Build history of the part. All positions in model axes, mm. Round coordinates to 2 decimals unless told otherwise and drop trailing zeros. Write each loop counter-clockwise with the first axis right and the second up, starting at its lowest first coordinate (ties: lowest second). Pieces come first, ordered by that corner, then holes.
1) Wall check: probe 1 along X at (y, z) = (30, 2); probe 2 along Y at (x, z) = (133.5, 4.25); probe 3 along X at (y, z) = (9.5, 0.5). Give the ranges that are in metal, low to high.
2) Flat gauge pins, fed straight in: pin 1 (9 mm diameter, centred on x = 127, y = 31.75, fed in from -Z); pin 2 (2 mm diameter, centred on x = 98.425, z = 5.08, fed in from +Y). Where does each tip first touch, or does it go through?
3) Pull direction Y, two halves, no side cores. Call faces 1 (the cylindrical face through (23.93, 51.16, 4.7)), 2 (the flat face through (69, 0, 5)), 3 (the cylindrical face through (98.501, 57.061, 6.806)): +Y half, -Y half, draft (parallel to the pull), parting line (faces both ways), or undercut.
4) Saw through at C-C (x = 25.4). Write the cut outline in (y, z) (3 decimals).
5) Saw through at B-B (z = 2). Write the cut outline in (x, y) (3 decimals).
6) Saw through at D-D (x = 94.5). Write the cut outline in (y, z) (3 decimals).
7) Saw through at A-A (x = 78.74). Write the cut outline in (y, z) (3 decimals).
from build123d import *

# Parameters (mm, degrees)
SKETCH1_W                   = 139.7
SKETCH1_H                   = 63.5
BOSS_EXTRUDE1_DEPTH         = 9.525
F_5_8_18_TAPPED_HOLE1_D     = 14.68374
F_1_4_0_25_DIAMETER_HOLE1_D = 6.35
F_8_32_TAPPED_HOLE1_D       = 3.4544
F_8_32_TAPPED_HOLE1_DEPTH   = 12.7
F_8_32_TAPPED_HOLE1_TIP     = 1.037806461
SKETCH9_R                   = 3.175
CUT_EXTRUDE1_DEPTH          = 10.525


with BuildPart() as part:
    # Sketch1 → Boss-Extrude1 (new body)
    with BuildSketch(Plane.XY):
        with Locations((69.85, 31.75)):
            Rectangle(SKETCH1_W, SKETCH1_H)
    extrude(amount=BOSS_EXTRUDE1_DEPTH)

    # 5/8-18 Tapped Hole1 (through all)
    with Locations(Plane.XY.offset(9.525)):
        with Locations((127, 31.75)):
            Hole(F_5_8_18_TAPPED_HOLE1_D / 2)

    # 1/4 (0.25) Diameter Hole1 (through all)
    with Locations(Plane(origin=(25.4, 53.975, 9.525), x_dir=(1, 0, 0), z_dir=(0, 0, 1))):
        with Locations((0, 0), (0, -44.45)):
            Hole(F_1_4_0_25_DIAMETER_HOLE1_D / 2)

    # #8-32 Tapped Hole1
    with Locations(Plane(origin=(98.425, 63.5, 5.08), x_dir=(0, 0, 1), z_dir=(0, 1, 0))):
        with Locations((0, 0)):
            Hole(F_8_32_TAPPED_HOLE1_D / 2, depth=F_8_32_TAPPED_HOLE1_DEPTH)
            with Locations((0, 0, -(F_8_32_TAPPED_HOLE1_DEPTH + F_8_32_TAPPED_HOLE1_TIP / 2))):  # 118° drill point
                Cone(0, F_8_32_TAPPED_HOLE1_D / 2, F_8_32_TAPPED_HOLE1_TIP, mode=Mode.SUBTRACT)

    # Sketch9 → Cut-Extrude1 (cut, through all)
    with BuildSketch(Plane.XY.offset(9.525)):
        with Locations((95.25, 31.75)):
            Circle(SKETCH9_R)
        with Locations((78.74, 31.75)):
            Circle(SKETCH9_R)
    extrude(amount=-CUT_EXTRUDE1_DEPTH, mode=Mode.SUBTRACT)


solid = part.part
Evaluation:
1. probe 1: x = 0 to 76.09, 81.39 to 92.6, 97.9 to 119.87, 134.13 to 139.7
1. probe 2: y = 0 to 28.34, 35.16 to 63.5
1. probe 3: x = 0 to 22.23, 28.57 to 139.7
2. pin 1: passes through
2. pin 2: stops at y = 50.36
3. face 1: undercut
3. face 2: -Y half
3. face 3: draft
4. outline: (0, 0) - (6.35, 0) - (6.35, 9.525) - (0, 9.525) - close; (12.7, 0) - (50.8, 0) - (50.8, 9.525) - (12.7, 9.525) - close; (57.15, 0) - (63.5, 0) - (63.5, 9.525) - (57.15, 9.525) - close
5. outline: (0, 0) - (139.7, 0) - (139.7, 63.5) - (0, 63.5) - close; hole circle Ø6.35 at (25.4, 9.525); hole circle Ø6.35 at (25.4, 53.975); hole circle Ø6.35 at (78.74, 31.75); hole circle Ø6.35 at (95.25, 31.75); hole circle Ø14.684 at (127, 31.75)
6. outline: (0, 0) - (28.665, 0) - (28.665, 9.525) - (0, 9.525) - close; (34.835, 0) - (63.5, 0) - (63.5, 9.525) - (34.835, 9.525) - close
7. outline: (0, 0) - (28.575, 0) - (28.575, 9.525) - (0, 9.525) - close; (34.925, 0) - (63.5, 0) - (63.5, 9.525) - (34.925, 9.525) - close
